Geometry: final body of the model. Coordinates: model frame, mm. Face numbers are marked on the shaded views. A direction names the side the tool comes from. Give positions to 0.01 mm unless a question says otherwise; leave off trailing zeros. Write each loop counter-clockwise with the first axis right and the second up, starting at its lowest first coordinate (ties: lowest second). Pieces come first, ordered by that corner, then holes. Notation, with made-up numbers: (36, 79.25) -> (83, 79.25) arc R23 cw to (83, 106.25) -> close; hole circle Ø6 at (-1.5, -19.5). An arc over 180 degrees is marked (long way). Use CSV: the item, a comma, the result in double quotes. Start each with the question number.
1) Contact query for flat-ended pins moving along their axis: P1, Ø3, axis at y = 4, z = 2, coming from the +X side; P2, Ø3, axis at x = 0, z = -1, coming from the -Y side; P3, Ø3, axis at y = 17.5, z = 2, coming from the -X side; P4, Ø1, axis at x = 2.5, z = 2, coming from the +Y side. Output: stop coordinate, or through.
2) Set-up query: the marked faces 1 and 2. Return all of +Z, -Z, +X, -X, +Y, -Y with unobstructed straight access to the full face (end or side cutting, diameter ignored); none if empty.
3) Section A-A (y = 23). Output: boundary loops of the cut face in (x, z), plus the area to 3 significant figures.
4) Material intervals for line 1 (Z direction, x = -1.75, y = 25.5); line 2 (Y direction, x = 2.25, z = -2.75); line 3 (Y direction, x = 0.5, z = 3.5), sorted ascending. Write a range as [from, to].
```python
from build123d import *

# Parameters (mm, degrees)
SKETCH1_R                   = 4
BOSS_EXTRUDE1_DEPTH         = 2
SKETCH2_R                   = 2.5
BOSS_EXTRUDE2_DEPTH         = 25
M2_TAPPED_HOLE1_D           = 1.6
M2_TAPPED_HOLE1_DEPTH       = 8
M2_TAPPED_HOLE1_CSINK_D     = 2.05
M2_TAPPED_HOLE1_CSINK_ANGLE = 90
M2_TAPPED_HOLE1_TIP         = 0.480688495
CHAMFER1_SIZE               = 1


with BuildPart() as part:
    # Sketch1 → Boss-Extrude1 (new body)
    with BuildSketch(Plane(origin=(0, 0, 0), x_dir=(1, 0, 0), z_dir=(0, 1, 0))):
        with Locations(Location((0, 0, 0), (0, 0, 270))):
            Circle(SKETCH1_R)
    extrude(amount=BOSS_EXTRUDE1_DEPTH)

    # Sketch2 → Boss-Extrude2 (add)
    with BuildSketch(Plane(origin=(0, 2, 0), x_dir=(1, 0, 0), z_dir=(0, 1, 0))):
        with Locations(Location((0, 0, 0), (0, 0, 270))):
            Circle(SKETCH2_R)
    extrude(amount=BOSS_EXTRUDE2_DEPTH)

    # M2 Tapped Hole1
    with Locations(Plane(origin=(0, 0, 0), x_dir=(-1, 0, 0), z_dir=(0, -1, 0))):
        with Locations((0, 0)):
            CounterSinkHole(M2_TAPPED_HOLE1_D / 2, M2_TAPPED_HOLE1_CSINK_D / 2, depth=M2_TAPPED_HOLE1_DEPTH, counter_sink_angle=M2_TAPPED_HOLE1_CSINK_ANGLE)
            with Locations((0, 0, -(M2_TAPPED_HOLE1_DEPTH + M2_TAPPED_HOLE1_TIP / 2))):  # 118° drill point
                Cone(0, M2_TAPPED_HOLE1_D / 2, M2_TAPPED_HOLE1_TIP, mode=Mode.SUBTRACT)

    # Chamfer1
    chamfer1_edges = [part.edges().sort_by_distance(p)[0] for p in [
        (0, 0, -4),
    ]]
    chamfer(chamfer1_edges, length=CHAMFER1_SIZE)


solid = part.part
```
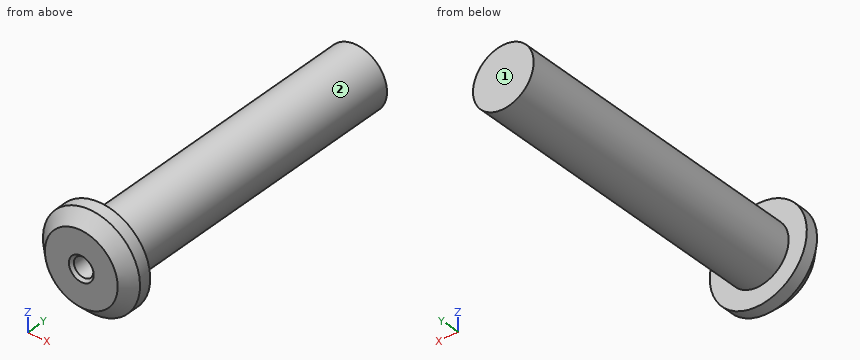
Answers follow:
1,P1,"stops at x = 2.45"
1,P2,"stops at y = 0"
1,P3,"stops at x = -2.45"
1,P4,"stops at y = 2"
2,face 1,"+Z, -Z, +X, -X, +Y"
2,face 2,"+Y"
3,outline,"circle Ø5 at (0, 0)"
3,area,"19.6 mm^2"
4,line 1,"z = [-1.79, 1.79]"
4,line 2,"y = [0.55, 2]"
4,line 3,"y = [0.54, 2]"
